Design review of the part built by this model. Coordinates are the model's own, in mm. A direction names the side the tool comes from. Give positions to 0.01 mm unless a question says otherwise; leave off trailing zeros. Order: outer loops, then holes, each group sorted by start corner. A loop starts at its lowest first (then second) coordinate and runs counter-clockwise, first axis right, second up.
```python
from build123d import *

# Parameters (mm, degrees)
SKETCH_1_W                   = 330
SKETCH_1_H                   = 200
EXTRUDE_1_DEPTH              = 12
SKETCH_2_W                   = 78.6
SKETCH_2_H                   = 2
CUT_EXTRUDE_1_DEPTH          = 387.062171159
SKETCH_4_R                   = 2.5
CUT_EXTRUDE_3_DEPTH          = 12
HOLE_WIZARD_M4_1_D           = 3.3
HOLE_WIZARD_M4_1_DEPTH       = 10.1
HOLE_WIZARD_M4_1_TIP         = 0.991420021
HOLE_WIZARD_M6_1_D           = 7
HOLE_WIZARD_M6_1_CBORE_D     = 11
HOLE_WIZARD_M6_1_CBORE_DEPTH = 6
HOLE_WIZARD_M3_1_D           = 3.6
HOLE_WIZARD_M3_1_CBORE_D     = 6.5
HOLE_WIZARD_M3_1_CBORE_DEPTH = 3
SKETCH_11_W                  = 60
SKETCH_11_H                  = 13
CUT_EXTRUDE_4_DEPTH          = 387.062171159
FILLET_1_R                   = 3
HOLE_WIZARD_M4_2_D           = 3.3
HOLE_WIZARD_M4_2_DEPTH       = 10.1
HOLE_WIZARD_M4_2_TIP         = 0.991420021
HOLE_WIZARD_M4_4_D           = 3.3
HOLE_WIZARD_M4_4_DEPTH       = 10.1
HOLE_WIZARD_M4_4_TIP         = 0.991420021
HOLE_WIZARD_M4_5_D           = 3.3
HOLE_WIZARD_M4_5_DEPTH       = 10.1
HOLE_WIZARD_M4_5_TIP         = 0.991420021


with BuildPart() as part:
    # 草图1 → 凸台-拉伸1 (new body)
    with BuildSketch(Plane.XY):
        with Locations((165, 100)):
            Rectangle(SKETCH_1_W, SKETCH_1_H)
    extrude(amount=EXTRUDE_1_DEPTH)

    # 草图2 → 切除-拉伸1 (cut, through all)
    with BuildSketch(Plane.XZ):
        with Locations((39.3, 1)):
            Rectangle(SKETCH_2_W, SKETCH_2_H)
        with Locations((290.7, 1)):
            Rectangle(SKETCH_2_W, SKETCH_2_H)
    extrude(amount=-CUT_EXTRUDE_1_DEPTH, mode=Mode.SUBTRACT)

    # 草图4 → 切除-拉伸3 (cut)
    with BuildSketch(Plane(origin=(0, 200, 0), x_dir=(1, 0, 0), z_dir=(0, 1, 0))):
        with Locations(Location((215, -6, 0), (0, 0, 270))):
            Circle(SKETCH_4_R)
    extrude(amount=-CUT_EXTRUDE_3_DEPTH, mode=Mode.SUBTRACT)

    # M4 螺纹孔1
    with Locations(Plane.XY.offset(12)):
        with Locations((109, 173), (131, 173), (199, 173), (221, 173), (21.5, 111), (21.5, 89), (59, 27), (81, 27), (249, 27), (271, 27), (304, 52), (304, 67), (304, 133), (304, 148)):
            Hole(HOLE_WIZARD_M4_1_D / 2, depth=HOLE_WIZARD_M4_1_DEPTH)
            with Locations((0, 0, -(HOLE_WIZARD_M4_1_DEPTH + HOLE_WIZARD_M4_1_TIP / 2))):  # 118° drill point
                Cone(0, HOLE_WIZARD_M4_1_D / 2, HOLE_WIZARD_M4_1_TIP, mode=Mode.SUBTRACT)

    # M6 六角凹头螺钉的柱形沉头孔1 (through all)
    with Locations(Plane.XY.offset(12)):
        with Locations((188, 167.5), (142, 167.5)):
            CounterBoreHole(HOLE_WIZARD_M6_1_D / 2, HOLE_WIZARD_M6_1_CBORE_D / 2, HOLE_WIZARD_M6_1_CBORE_DEPTH)

    # M3 六角凹头螺钉的柱形沉头孔1 (through all)
    with Locations(Plane.XY.offset(12)):
        with Locations((70, 150), (50, 150), (50, 130), (70, 130), (70, 50), (50, 50), (70, 70), (50, 70), (280, 50), (260, 50), (280, 70), (260, 70), (280, 150), (260, 150), (280, 130), (260, 130)):
            CounterBoreHole(HOLE_WIZARD_M3_1_D / 2, HOLE_WIZARD_M3_1_CBORE_D / 2, HOLE_WIZARD_M3_1_CBORE_DEPTH)

    # 草图11 → 切除-拉伸4 (cut, through all)
    with BuildSketch(Plane.XY.offset(12)):
        with Locations((105, 193.5)):
            Rectangle(SKETCH_11_W, SKETCH_11_H)
        with Locations((105, 6.5)):
            Rectangle(SKETCH_11_W, SKETCH_11_H)
    extrude(amount=-CUT_EXTRUDE_4_DEPTH, mode=Mode.SUBTRACT)

    # 圆角1
    fillet_1_edges = [part.edges().sort_by_distance(p)[0] for p in [
        (75, 187, 7),
        (135, 187, 6),
        (75, 200, 7),
        (135, 200, 6),
        (75, 0, 7),
        (135, 0, 6),
        (75, 13, 7),
        (135, 13, 6),
    ]]
    fillet(fillet_1_edges, radius=FILLET_1_R)

    # M4 螺纹孔2
    with Locations(Plane.XY.offset(12)):
        with Locations((215, 195)):
            Hole(HOLE_WIZARD_M4_2_D / 2, depth=HOLE_WIZARD_M4_2_DEPTH)
            with Locations((0, 0, -(HOLE_WIZARD_M4_2_DEPTH + HOLE_WIZARD_M4_2_TIP / 2))):  # 118° drill point
                Cone(0, HOLE_WIZARD_M4_2_D / 2, HOLE_WIZARD_M4_2_TIP, mode=Mode.SUBTRACT)

    # M4 螺纹孔4
    with Locations(Plane(origin=(0, 0, 2), x_dir=(-1, 0, 0), z_dir=(0, 0, -1))):
        with Locations((-299.5, 167), (-299.5, 157), (-299.5, 103), (-299.5, 93)):
            Hole(HOLE_WIZARD_M4_4_D / 2, depth=HOLE_WIZARD_M4_4_DEPTH)
            with Locations((0, 0, -(HOLE_WIZARD_M4_4_DEPTH + HOLE_WIZARD_M4_4_TIP / 2))):  # 118° drill point
                Cone(0, HOLE_WIZARD_M4_4_D / 2, HOLE_WIZARD_M4_4_TIP, mode=Mode.SUBTRACT)

    # M4 螺纹孔5
    with Locations(Plane(origin=(0, 0, 0), x_dir=(-1, 0, 0), z_dir=(0, 0, -1))):
        with Locations((-89.5, 158), (-89.5, 168), (-89.5, 93), (-89.5, 103)):
            Hole(HOLE_WIZARD_M4_5_D / 2, depth=HOLE_WIZARD_M4_5_DEPTH)
            with Locations((0, 0, -(HOLE_WIZARD_M4_5_DEPTH + HOLE_WIZARD_M4_5_TIP / 2))):  # 118° drill point
                Cone(0, HOLE_WIZARD_M4_5_D / 2, HOLE_WIZARD_M4_5_TIP, mode=Mode.SUBTRACT)


solid = part.part
```
1. Take a section at B-B (x = 95). State the section outline as (y, z) points, then the cut area to 3 significant figures.
Recorded:
outline: (13, 0) - (187, 0) - (187, 12) - (13, 12) - close
area: 2,090 mm2
2. Take a section at C-C (x = 43). State the section outline as (y, z) points.
Recorded:
outline: (0, 2) - (200, 2) - (200, 12) - (0, 12) - close
3. Machinability: for faces 3 (the face through (281.4, 148.6, 9)), 4 (the face through (35, 200, 7)), 5 (the face through (105, 187, 6)), which of the approach directions +Z, -Z, +X, -X, +Y, -Y give a long, thin tool a straight path to every point of the face, cutting with its end or side? Answer none if there is none.
Recorded:
face 3: +Z
face 4: +Z, -Z, +X, -X, +Y
face 5: +Z, -Z, +Y
4. For line 1 along X through (y, z) = (130, 10.5); line 2 along Y through (x, z) = (280, 6); line 3 along Y through (x, z) = (50, 11.3), list the stretches that pass through material, from the lowest coordinate up.
Recorded:
line 1: x = 0 to 46.75, 53.25 to 66.75, 73.25 to 256.75, 263.25 to 276.75, 283.25 to 330
line 2: y = 0 to 48.2, 51.8 to 68.2, 71.8 to 128.2, 131.8 to 148.2, 151.8 to 200
line 3: y = 0 to 46.75, 53.25 to 66.75, 73.25 to 126.75, 133.25 to 146.75, 153.25 to 200
5. Draft analysis for pull direction X (two halves, no side actions). For faces 1 (the face through (277.421, 48.022, 10.521)), 2 (the face through (35, 0, 7)), state which applies: pulls with the +X half, pulls with the -X half, needs draft (parallel to the pull), parting line crosses it, or undercut.
Recorded:
face 1: undercut
face 2: needs draft
6. Take a section at A-A (y = 140.5). State the section outline as (x, z) points.
Recorded:
outline: (0, 2) - (78.6, 2) - (78.6, 0) - (251.4, 0) - (251.4, 2) - (330, 2) - (330, 12) - (0, 12) - close
7. For pin 1 (10.5 mm diameter, centred on x = 70, y = 150, fed in from -Z); pin 2 (4 mm diameter, centred on x = 108.5, z = 7, fed in from +Y); pin 3 (4 mm diameter, centred on x = 70, y = 50, fed in from +Z), all flat-tipped, find the tip position at first contact; note any pin that passes through.
Recorded:
pin 1: stops at z = 2
pin 2: stops at y = 187
pin 3: stops at z = 9
